from build123d import *

# Parameters (mm, degrees)
F1_DEPTH = 666
F3_DEPTH = 2


with BuildPart() as f1:
    # F0 (on Top) → F1 (new body)
    with BuildSketch(Plane.XY):
        with BuildLine():
            Line((46.156122, 23.872672), (-51.843878, 23.872672))
            ThreePointArc((-51.843878, 23.872672), (-52.550985, 23.579779), (-52.843878, 22.872672))
            Line((-52.843878, 22.872672), (-52.843878, 5.772672))
            ThreePointArc((-52.843878, 5.772672), (-52.550985, 5.065565), (-51.843878, 4.772672))
            Line((-51.843878, 4.772672), (-42.843878, 4.772672))
            Line((-42.843878, 4.772672), (-42.843878, 6.772672))
            Line((-42.843878, 6.772672), (-49.843878, 6.772672))
            ThreePointArc((-49.843878, 6.772672), (-50.550985, 7.065565), (-50.843878, 7.772672))
            Line((-50.843878, 7.772672), (-50.843878, 20.872672))
            ThreePointArc((-50.843878, 20.872672), (-50.550985, 21.579779), (-49.843878, 21.872672))
            Line((-49.843878, 21.872672), (44.156122, 21.872672))
            ThreePointArc((44.156122, 21.872672), (44.863229, 21.579779), (45.156122, 20.872672))
            Line((45.156122, 20.872672), (45.156122, 7.772672))
            ThreePointArc((45.156122, 7.772672), (44.863229, 7.065565), (44.156122, 6.772672))
            Line((44.156122, 6.772672), (36.389313, 6.772672))
            Line((36.389313, 6.772672), (36.389313, 4.772672))
            Line((36.389313, 4.772672), (46.156122, 4.772672))
            ThreePointArc((46.156122, 4.772672), (46.863229, 5.065565), (47.156122, 5.772672))
            Line((47.156122, 5.772672), (47.156122, 22.872672))
            ThreePointArc((47.156122, 22.872672), (46.863229, 23.579779), (46.156122, 23.872672))
        make_face()
    extrude(amount=F1_DEPTH)

    # F2 (on face) → F3 (cut, through all)
    with BuildSketch(Plane.XZ.offset(-21.872672)):
        with BuildLine():
            ThreePointArc((-32.843878, 64), (-2.843878, 34), (27.156122, 64))
            Line((27.156122, 64), (27.156122, 194))
            ThreePointArc((27.156122, 194), (-2.843878, 224), (-32.843878, 194))
            Line((-32.843878, 194), (-32.843878, 64))
        make_face()
    extrude(amount=-F3_DEPTH, mode=Mode.SUBTRACT)


solid = f1.part
Geometry check sheet. Reference: the model listing, model coordinates, mm. A direction names the side the tool comes from. Give positions to 0.01 mm unless a question says otherwise; leave off trailing zeros. Loops run counter-clockwise (first coordinate to the right, second up) from the corner with the lowest first, then second, coordinate; pieces in that order, holes last. Notation, with made-up numbers: M -2.5,-39 L 21.5,-39 A26 cw 21.5,-1 Z; hole C 44,7.25 d11. An arc over 180 degrees is marked long. Write each question's results on one line, items separated by ' | '.
1) Gauge pin test, flat end, axial feed: pin 1 (10 mm diameter, centred on x = 14, z = 363.5, fed in from -Y). Record the tip position at first contact, or that the pin passes through.
Answers follow:
pin 1: y = 21.87
2) Thickness scan on line 1 (X direction, y = 17.25, z = 35); line 2 (Y direction, x = 38.5, z = 79); line 3 (Y direction, x = 3, z = 293). Record the ranges inside material, lowest first.
Answers follow:
line 1: -52.84 to -50.84, 45.16 to 47.16 | line 2: 4.77 to 6.77, 21.87 to 23.87 | line 3: 21.87 to 23.87
3) Release check for a two-part mould opening along Y. For faces 1 (the face through (47.156, 14, 328)), 2 (the face through (-50.844, 14, 328)), 3 (the face through (-4, 21.873, 328)), 4 (the face through (-2, 23.873, 328)) record: +Y half, -Y half, draft (parallel to the pull), parting line (faces both ways), or undercut.
Answers follow:
face 1: draft | face 2: undercut | face 3: undercut | face 4: +Y half
4) Section check C-C, the plane x = 5. Record the boundary of the cut face in (y, z), plus the area to 3 significant figures.
Answers follow:
outline: M 21.87,0 L 23.87,0 L 23.87,35.04 L 21.87,35.04 Z; M 21.87,222.96 L 23.87,222.96 L 23.87,666 L 21.87,666 Z | area: 956 mm2
5) Section check A-A, the plane z = 93. Record the boundary of the cut face in (x, y), plus the area to 3 significant figures.
Answers follow:
outline: M -52.84,5.77 A1 ccw -51.84,4.77 L -42.84,4.77 L -42.84,6.77 L -49.84,6.77 A1 cw -50.84,7.77 L -50.84,20.87 A1 cw -49.84,21.87 L -32.84,21.87 L -32.84,23.87 L -51.84,23.87 A1 ccw -52.84,22.87 Z; M 27.16,21.87 L 44.16,21.87 A1 cw 45.16,20.87 L 45.16,7.77 A1 cw 44.16,6.77 L 36.39,6.77 L 36.39,4.77 L 46.16,4.77 A1 ccw 47.16,5.77 L 47.16,22.87 A1 ccw 46.16,23.87 L 27.16,23.87 Z | area: 182 mm2
6) Section check B-B, the plane y = 17.25. Record the boundary of the cut face in (x, z).
Answers follow:
outline: M -52.84,0 L -50.84,0 L -50.84,666 L -52.84,666 Z; M 45.16,0 L 47.16,0 L 47.16,666 L 45.16,666 Z
7) Tool access check on faces 5 (the face through (-52.844, 14, 328)), 6 (the face through (45.156, 14, 328)), 7 (the face through (-2.184, 22.859, 223.993)). Record the directions out of +Z, -Z, +X, -X, +Y, -Y that give a thin tool (end or side, any length) a straight path to the whole face; none if there is none.
Answers follow:
face 5: +Z, -Z, -X, +Y, -Y | face 6: +Z, -Z | face 7: +Y, -Y
8) Section check D-D, the plane z = 394. Record the boundary of the cut face in (x, y).
Answers follow:
outline: M -52.84,5.77 A1 ccw -51.84,4.77 L -42.84,4.77 L -42.84,6.77 L -49.84,6.77 A1 cw -50.84,7.77 L -50.84,20.87 A1 cw -49.84,21.87 L 44.16,21.87 A1 cw 45.16,20.87 L 45.16,7.77 A1 cw 44.16,6.77 L 36.39,6.77 L 36.39,4.77 L 46.16,4.77 A1 ccw 47.16,5.77 L 47.16,22.87 A1 ccw 46.16,23.87 L -51.84,23.87 A1 ccw -52.84,22.87 Z
